Verification items for the finished model (mm, model axes). A direction names the side the tool comes from. Coordinates: 2 decimals unless noted, no trailing zeros. Order: outer loops, then holes, each group sorted by start corner. A loop starts at its lowest first (then second) coordinate and runs counter-clockwise, first axis right, second up. Notation, with made-up numbers: M -15.5,47 L -7.5,47 A20 ccw -7.5,60 Z; hole C 81.25,1.5 d9. An arc over 180 degrees is marked long. Return JSON: item names as keys, results as strings. Group by question number.
1. Set-up check for faces 1 (the cylindrical face through (-9.66, -0.37, -2.53)), 2 (the cylindrical face through (0, -3, -16)): record each of +Z, -Z, +X, -X, +Y, -Y from which the full face is reachable in a straight line by a thin tool's end or side.
2. Gauge pin test, flat ends, axial feed: pin 1 (1.5 mm diameter, centred on y = -2.5, z = -14, fed in from -X); pin 2 (10 mm diameter, centred on x = 9.5, y = 0, fed in from -Z); pin 3 (6 mm diameter, centred on y = 5, z = -5.5, fed in from -X). Record the tip position at first contact, or that the pin passes through.
3. Mould release check, pull along X, two halves, no side actions. Record for faces 3 (the cylindrical face through (-0.37, 9.66, -2.53)), 4 (the flat face through (0, 0, 0)), 5 (the cylindrical face through (9.66, 0.37, -2.53)), 6 (the cylindrical face through (-3.755, 11.923, -2.521)): +X half, -X half, draft (parallel to the pull), parting line (faces both ways), or undercut.
4. Section check A-A, the plane x = 0. Record the cut outline in (y, z).
5. Section check B-B, the plane z = -24. Record the cut outline in (x, y), plus the area to 3 significant figures.
6. Material ranges on line 1 along X through (y, z) = (0, -1.1); line 2 along Z through (x, y) = (7.75, -7.5), recorded low to high.
```python
from build123d import *

# Parameters (mm, degrees)
M3_CLEARANCE_HOLE1_D = 3.4
CIRPATTERN1_COUNT    = 4
CHAMFER1_SIZE        = 1


with BuildPart() as part:
    # Sketch1 → Revolve1 (revolve)
    with BuildSketch(Plane(origin=(0, 0, 0), x_dir=(0, 0, -1), z_dir=(1, 0, 0))):
        Polygon((0, 0), (0, 12.5), (5, 12.5), (5, 3), (27, 3), (27, 0), align=None)
    revolve(axis=Axis((0, 0, -27), (0, 0, 1)))

    # M3 Clearance Hole1 (through all)
    with Locations(Plane(origin=(8, 0, 0), x_dir=(0, 1, 0), z_dir=(0, 0, 1))):
        with Locations((0, 0)):
            m3_clearance_hole1 = Hole(M3_CLEARANCE_HOLE1_D / 2)

    # CirPattern1: M3 Clearance Hole1 ×4 about axis
    cirpattern1_axis = Axis((0, 0, 0), (0, 0, 1))
    for i in range(1, CIRPATTERN1_COUNT):
        add(m3_clearance_hole1.rotate(cirpattern1_axis, i * 360 / CIRPATTERN1_COUNT), mode=Mode.SUBTRACT)

    # Chamfer1
    chamfer1_edges = [part.edges().sort_by_distance(p)[0] for p in [
        (0, -12.5, -5),
        (0, -12.5, 0),
    ]]
    chamfer(chamfer1_edges, length=CHAMFER1_SIZE)


solid = part.part
```
Answers follow:
{
 "1": {"face 1": "+Z, -Z", "face 2": "-Z"},
 "2": {"pin 1": "x = -2.44", "pin 2": "z = -5", "pin 3": "x = -12.27"},
 "3": {"face 3": "undercut", "face 4": "draft", "face 5": "undercut", "face 6": "parting line"},
 "4": {"outline": "M -12.5,-4 L -11.5,-5 L -9.7,-5 L -9.7,0 L -11.5,0 L -12.5,-1 Z; M -6.3,-5 L -3,-5 L -3,-27 L 3,-27 L 3,-5 L 6.3,-5 L 6.3,0 L -6.3,0 Z; M 9.7,-5 L 11.5,-5 L 12.5,-4 L 12.5,-1 L 11.5,0 L 9.7,0 Z"},
 "5": {"outline": "C 0,0 d6", "area": "28.3 mm^2"},
 "6": {"line 1": "-12.5 to -9.7, -6.3 to 6.3, 9.7 to 12.5", "line 2": "-5 to 0"}
}
